The model under review builds one solid part; all positions refer to its coordinate system, in mm. Coordinates: 2 decimals unless noted, no trailing zeros. Order: outer loops, then holes, each group sorted by start corner. A loop starts at its lowest first (then second) coordinate and runs counter-clockwise, first axis right, second up. Notation, with made-up numbers: M 33.25,56.25 L 42.25,56.25 A17 cw 42.25,64.25 Z; hole C 42.5,42.25 d1. An arc over 180 degrees is marked long. Answer in a Markdown table with one row per item.
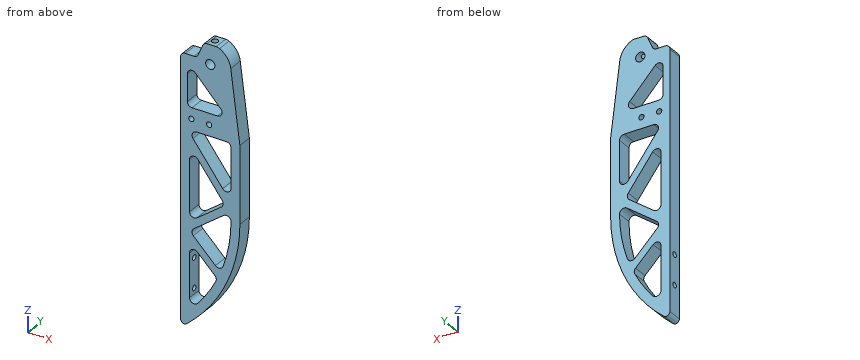
from build123d import *
from OCP.BRepFilletAPI import BRepFilletAPI_MakeFillet

# Parameters (mm, degrees)
SKETCH1_W                      = 50.8
SKETCH1_H                      = 243.84
BOSS_EXTRUDE1_DEPTH            = 6.35
SKETCH2_R                      = 4
PIVOT_POINT_DEPTH              = 126.183610748
MAIN_SHAPE_DEPTH               = 126.183610748
OPTIMIZING_WEIGHT_CUTOUT_DEPTH = 126.183610748
F_8_CLEARANCE_HOLE1_REACH      = 134.233
F_8_CLEARANCE_HOLE1_BORE_R     = 2.2479
F_1_4_28_TAPPED_HOLE1_D        = 5.4102
F_1_4_28_TAPPED_HOLE1_DEPTH    = 13.97
F_1_4_28_TAPPED_HOLE1_TIP      = 1.625388061
FILLET1_R1                     = 3.96875
FILLET1_R2                     = 3.175
F_8_CLEARANCE_HOLE2_D          = 4.4958


with BuildPart() as part:
    # Sketch1 → Boss-Extrude1 (new, symmetric)
    with BuildSketch(Plane(origin=(0, 0, 0), x_dir=(1, 0, 0), z_dir=(0, 1, 0))):
        Rectangle(SKETCH1_W, SKETCH1_H)
    extrude(amount=BOSS_EXTRUDE1_DEPTH, both=True)

    # Sketch2 → Pivot Point (cut, through all)
    with BuildSketch(Plane(origin=(0, 6.35, 0), x_dir=(1, 0, 0), z_dir=(0, 1, 0))):
        with Locations(Location((0, -105.41, 0), (0, 0, 270))):
            Circle(SKETCH2_R)
    extrude(amount=-PIVOT_POINT_DEPTH, mode=Mode.SUBTRACT)

    # Sketch3 → Main Shape (cut, through all)
    with BuildSketch(Plane(origin=(0, 6.35, 0), x_dir=(1, 0, 0), z_dir=(0, 1, 0))):
        Polygon((-11.332366666, -107.95), (-25.4, -107.95), (-25.4, -121.92), (-5.402453483, -121.92), align=None)
        with BuildLine():
            Line((25.4, 121.92), (-25.4, 121.92))
            ThreePointArc((-25.4, 121.92), (11.992253257, 77.116126628), (25.4, 20.32))
            Line((25.4, 20.32), (25.4, 121.92))
        make_face()
        with BuildLine():
            Line((25.4, -121.92), (25.4, -45.72))
            Line((25.4, -45.72), (17.569250135, -107.632186158))
            ThreePointArc((17.569250135, -107.632186158), (14.449275969, -115.648900605), (7.919806331, -121.249612663))
            ThreePointArc((7.919806331, -121.249612663), (6.538931045, -121.750131083), (5.08, -121.92))
            Line((5.08, -121.92), (25.4, -121.92))
        make_face()
    extrude(amount=-MAIN_SHAPE_DEPTH, mode=Mode.SUBTRACT)

    # Sketch4 → Optimizing Weight Cutout (cut, through all)
    with BuildSketch(Plane(origin=(0, 6.35, 0), x_dir=(1, 0, 0), z_dir=(0, 1, 0))):
        with BuildLine():
            ThreePointArc((6.024131859, 71.978790555), (-4.436732062, 89.680534626), (-17.78, 105.324658696))
            Line((-17.78, 105.324658696), (-17.78, 48.174658696))
            Line((-17.78, 48.174658696), (6.024131859, 71.978790555))
        make_face()
        with BuildLine():
            Line((8.791407169, 65.765809744), (-17.78, 39.194402575))
            Line((-17.78, 39.194402575), (17.78, 12.524402575))
            Line((17.78, 12.524402575), (17.78, 20.32))
            ThreePointArc((17.78, 20.32), (15.511294476, 43.483097938), (8.791407169, 65.765809744))
        make_face()
        Polygon((12.7, 8.396902575), (-17.78, 31.256902575), (-17.78, -32.243097425), align=None)
        Polygon((17.78, -45.240017282), (17.78, 4.586902575), (-19.590189893, -45.240017282), align=None)
        Polygon((15.370526289, -64.290017282), (-19.590189893, -64.290017282), (-19.590189893, -101.6), align=None)
    extrude(amount=-OPTIMIZING_WEIGHT_CUTOUT_DEPTH, mode=Mode.SUBTRACT)

    # #8 Clearance Hole1 bore → #8 Clearance Hole1 (cut, up to next)
    with BuildSketch(Plane.ZY.offset(25.4), mode=Mode.PRIVATE) as f_8_clearance_hole1_sk1:
        with Locations((-90.17, 0)):
            Circle(F_8_CLEARANCE_HOLE1_BORE_R)
    f_8_clearance_hole1_tool1 = extrude(f_8_clearance_hole1_sk1.sketch, amount=-F_8_CLEARANCE_HOLE1_REACH, mode=Mode.PRIVATE) & part.part
    # #8 Clearance Hole1 bore → #8 Clearance Hole1 (cut, up to next)
    with BuildSketch(Plane.ZY.offset(25.4), mode=Mode.PRIVATE) as f_8_clearance_hole1_sk2:
        with Locations((-64.77, 0)):
            Circle(F_8_CLEARANCE_HOLE1_BORE_R)
    f_8_clearance_hole1_tool2 = extrude(f_8_clearance_hole1_sk2.sketch, amount=-F_8_CLEARANCE_HOLE1_REACH, mode=Mode.PRIVATE) & part.part
    add(f_8_clearance_hole1_tool1.solids().sort_by_distance((-25.4, 0, -90.17))[0], mode=Mode.SUBTRACT)
    add(f_8_clearance_hole1_tool2.solids().sort_by_distance((-25.4, 0, -64.77))[0], mode=Mode.SUBTRACT)

    # 1/4-28 Tapped Hole1
    with Locations(Plane.XY.offset(121.92)):
        with Locations((0, 0)):
            Hole(F_1_4_28_TAPPED_HOLE1_D / 2, depth=F_1_4_28_TAPPED_HOLE1_DEPTH)
            with Locations((0, 0, -(F_1_4_28_TAPPED_HOLE1_DEPTH + F_1_4_28_TAPPED_HOLE1_TIP / 2))):  # 118° drill point
                Cone(0, F_1_4_28_TAPPED_HOLE1_D / 2, F_1_4_28_TAPPED_HOLE1_TIP, mode=Mode.SUBTRACT)

    # Fillet1: one fillet with a radius per group of edges: ONE call of the kernel's fillet builder (fillet() takes one radius for all edges)
    fillet1_edges_1 = [part.edges().sort_by_distance(p)[0] for p in [
        (-17.78, 0, -39.194402575),
        (17.78, 0, -12.524402575),
        (-17.78, 0, -31.256902575),
        (8.791407169, 0, -65.765809744),
        (6.024131859, 0, -71.978790555),
        (-17.78, 0, -48.174658696),
        (-17.78, 0, -105.324658696),
        (-5.402453483, 0, 121.92),
        (-25.4, 0, 107.95),
        (-11.332366666, 0, 107.95),
        (-17.78, 0, 32.243097425),
        (12.7, 0, -8.396902575),
        (-19.590189893, 0, 45.240017282),
        (17.78, 0, -4.586902575),
        (17.78, 0, 45.240017282),
        (-19.590189893, 0, 101.6),
        (-19.590189893, 0, 64.290017282),
        (15.370526289, 0, 64.290017282),
    ]]
    fillet1_edges_2 = [part.edges().sort_by_distance(p)[0] for p in [
        (-25.4, 0, -121.92),
    ]]
    fillet1 = BRepFilletAPI_MakeFillet(part.part.solid().wrapped)
    for e in fillet1_edges_1:
        fillet1.Add(FILLET1_R1, e.wrapped)
    for e in fillet1_edges_2:
        fillet1.Add(FILLET1_R2, e.wrapped)
    add(Compound.cast(fillet1.Shape()), mode=Mode.REPLACE)

    # #8 Clearance Hole2 (through all)
    with Locations(Plane(origin=(0, 6.35, 0), x_dir=(1, 0, 0), z_dir=(0, 1, 0))):
        with Locations((-16.2052, -54.79148033), (-0.9652, -54.79148033)):
            Hole(F_8_CLEARANCE_HOLE2_D / 2)


solid = part.part
(1) Take a section at D-D (z = 32.5). Write out the cut boundary in (x, y), then the cut area to 3 significant figures.
Report:
| item | result |
|---|---|
| outline | M -25.4,-6.35 L -10.04,-6.35 L -10.04,6.35 L -25.4,6.35 Z; M 17.78,-6.35 L 25.4,-6.35 L 25.4,6.35 L 17.78,6.35 Z |
| area | 292 mm^2 |
(2) Take a section at A-A (z = -13.5). Write out the cut boundary in (x, y).
Report:
| item | result |
|---|---|
| outline | M -25.4,-6.35 L -17.78,-6.35 L -17.78,6.35 L -25.4,6.35 Z; M 5.9,-6.35 L 25.4,-6.35 L 25.4,6.35 L 5.9,6.35 Z |
(3) Take a section at B-B (z = -64.77). Write out the cut boundary in (x, y), then the cut area to 3 significant figures.
Report:
| item | result |
|---|---|
| outline | M -25.4,-6.35 L -17.78,-6.35 L -17.78,-2.25 L -25.4,-2.25 Z; M -25.4,2.25 L -17.78,2.25 L -17.78,6.35 L -25.4,6.35 Z; M -1.18,-6.35 L 17.37,-6.35 L 17.37,6.35 L -1.18,6.35 Z |
| area | 298 mm^2 |
(4) Insertion check: P1, Ø3.5, axis at y = 0, z = -64.77, coming from the +X side; P2, Ø5, axis at x = -14, y = 3.5, coming from the -Z side; P3, Ø6, axis at x = -16, y = 2.5, coming from the +Z side. Each pin has a flat end and moves straight along its axis. Give the tip position at first contact, or say it passes through.
Report:
| item | result |
|---|---|
| P1 | x = 18.01 |
| P2 | z = -114.59 |
| P3 | z = 108.07 |
(5) To check wall thickness, follow line 1 (Z direction, x = -18.5, y = 1); line 2 (Z direction, x = -12, y = 1.5); line 3 (Y direction, x = -20.75, z = -90.17). State the ranges of each line that lie inside material, in increasing order. Write a range as [from, to].
Report:
| item | result |
|---|---|
| line 1 | [-116.36, -92.18], [-88.16, -66.78], [-62.76, 65.53], [94.29, 107.95] |
| line 2 | [-110.32, -98.77], [-54.22, -44.97], [-34.86, -26.85], [23.87, 35.12], [45.22, 64.29], [93.5, 108.47] |
| line 3 | [-6.35, -2.25], [2.25, 6.35] |
(6) Take a section at C-C (y = 0). State how many separate pieces and enclosed holes the cut face has, then the cut area to 3 significant figures.
Report:
| item | result |
|---|---|
| separate pieces | 2 |
| enclosed holes | 6 |
| area | 5,950 mm^2 |
